Input: dimensioned drawing with shaded views. Units: mm. Origin: part minimum x, y, z. A direction names the side the tool comes from. Round coordinates to 2 decimals unless told otherwise and drop trailing zeros. Loops run counter-clockwise (first coordinate to the right, second up) from the corner with the lowest first, then second, coordinate; pieces in that order, holes last. Notation, with made-up numbers: (68, -17) - (89, -17) arc R17 cw to (89, 12) - close; hole circle Ø3 at (-1, 78). An arc over 180 degrees is marked (long way). Answer as CSV lines item,"result".
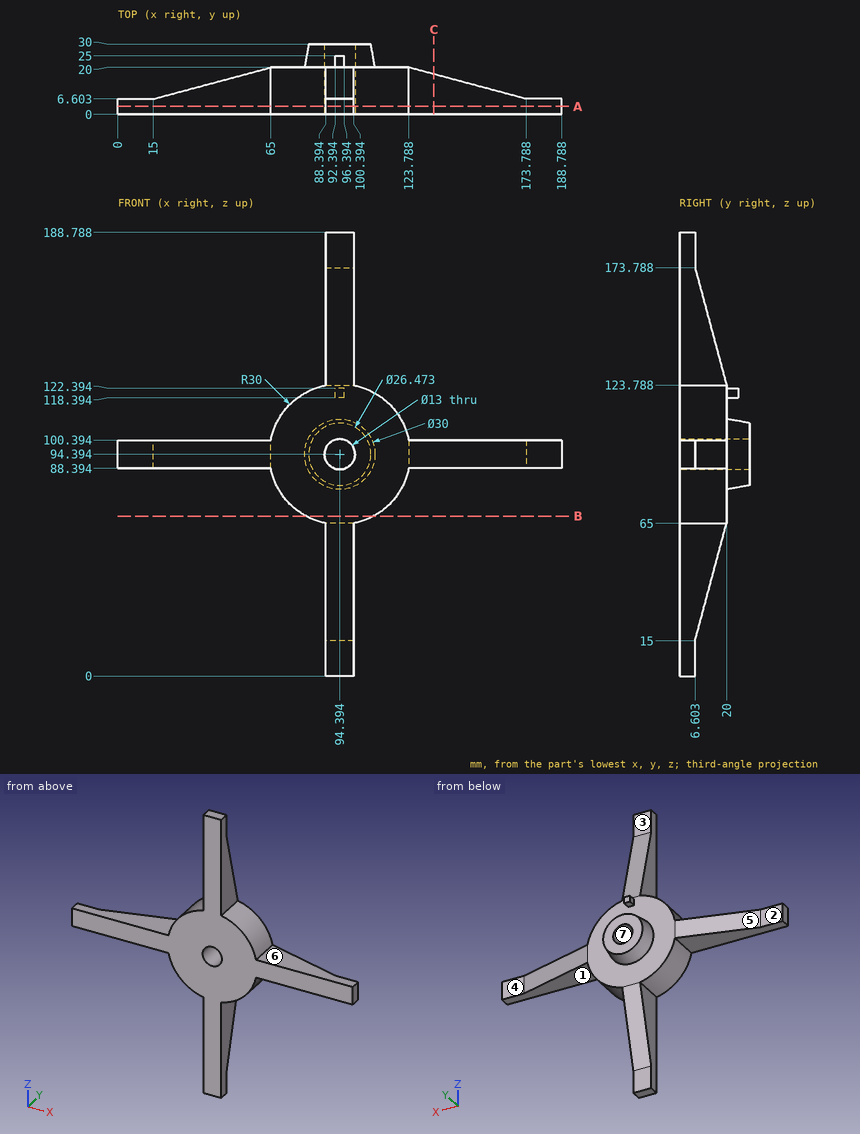
(1) Section A-A (y = 3.5). Output: boundary loops of the cut face in (x, z).
Findings below:
outline,"(0, 88.39) - (65, 88.39) arc R30 ccw to (88.39, 65) - (88.39, 0) - (100.39, 0) - (100.39, 65) arc R30 ccw to (123.79, 88.39) - (188.79, 88.39) - (188.79, 100.39) - (123.79, 100.39) arc R30 ccw to (100.39, 123.79) - (100.39, 188.79) - (88.39, 188.79) - (88.39, 123.79) arc R30 ccw to (65, 100.39) - (0, 100.39) - close; hole circle Ø13 at (94.39, 94.39)"
(2) Section B-B (z = 68). Output: boundary loops of the cut face in (x, y) (1 decimal).
Findings below:
outline,"(80.1, 0) - (108.7, 0) - (108.7, 20) - (80.1, 20) - close"
(3) Material intervals for line 1 along Z through (x, y) = (124, 5); line 2 along Y through (x, z) = (79, 93.5), sorted ascending.
Findings below:
line 1,"88.39 to 100.39"
line 2,"0 to 20"
(4) Pin query (flat end, axial travel): P1, Ø1, axis at x = 41, y = 8, coming from the +Z side; P2, Ø16, axis at x = 153, y = 6.5, coming from the -Z side; P3, Ø16, axis at y = 6.5, z = 48.5, coming from the -X side. Return the tip coordinate at first contact, or that it passes through.
Findings below:
P1,"z = 100.39"
P2,"z = 88.39"
P3,"x = 88.39"
(5) Section C-C (x = 134.5). Output: boundary loops of the cut face in (y, z), and give its area (3 significant figures).
Findings below:
outline,"(0, 88.39) - (17.13, 88.39) - (17.13, 100.39) - (0, 100.39) - close"
area,"206 mm2"
(6) Access query for the marked faces 1, 2, 3 and 4. Directions: +Z, -Z, +X, -X, +Y, -Y. A direction counts if a zero-diameter tool reaches every point of the face in a straight line with its end or side. Return the directions, or none.
Findings below:
face 1,"-Z, +X, +Y, -Y"
face 2,"+Z, -Z, -X, +Y"
face 3,"+Z, +X, -X, +Y"
face 4,"+Z, -Z, +X, +Y"
(7) Draft query along Z for the marked faces 5, 6 and 7. Return one class per face: pulls with the +Z half, pulls with the -Z half, needs draft (parallel to the pull), parting line crosses it, or undercut.
Findings below:
face 5,"needs draft"
face 6,"pulls with the +Z half"
face 7,"undercut"
